```python
from build123d import *

# Parameters (mm, degrees)
SKETCH1_W           = 380
SKETCH1_H           = 179
BOSS_EXTRUDE1_DEPTH = 20
SKETCH2_W           = 20
SKETCH2_H           = 65
SKETCH2_H_2         = 10
CUT_EXTRUDE1_DEPTH  = 20
SKETCH3_R           = 5
CUT_EXTRUDE2_DEPTH  = 159


with BuildPart() as part:
    # Sketch1 → Boss-Extrude1 (new body)
    with BuildSketch(Plane(origin=(0, 0, 0), x_dir=(0, 0, -1), z_dir=(1, 0, 0))):
        Rectangle(SKETCH1_W, SKETCH1_H)
    extrude(amount=BOSS_EXTRUDE1_DEPTH)

    # Sketch2 → Cut-Extrude1 (cut)
    with BuildSketch(Plane.XY.offset(190)):
        with Locations((10, 38)):
            Rectangle(SKETCH2_W, SKETCH2_H)
        with Locations((10, 84.5)):
            Rectangle(SKETCH2_W, SKETCH2_H_2)
        with Locations((10, -84.5)):
            Rectangle(SKETCH2_W, SKETCH2_H_2)
        with Locations((10, -37)):
            Rectangle(SKETCH2_W, SKETCH2_H)
    cut_extrude1 = extrude(amount=-CUT_EXTRUDE1_DEPTH, mode=Mode.SUBTRACT)

    # Sketch3 → Cut-Extrude2 (cut)
    with BuildSketch(Plane(origin=(0, 79.5, 0), x_dir=(1, 0, 0), z_dir=(0, 1, 0))):
        with Locations((10, -180)):
            Circle(SKETCH3_R)
    cut_extrude2 = extrude(amount=-CUT_EXTRUDE2_DEPTH, mode=Mode.SUBTRACT)

    # Mirror2: Cut-Extrude1, Cut-Extrude2 across plane
    add(cut_extrude1.mirror(Plane.XY), mode=Mode.SUBTRACT)
    add(cut_extrude2.mirror(Plane.XY), mode=Mode.SUBTRACT)


solid = part.part
```
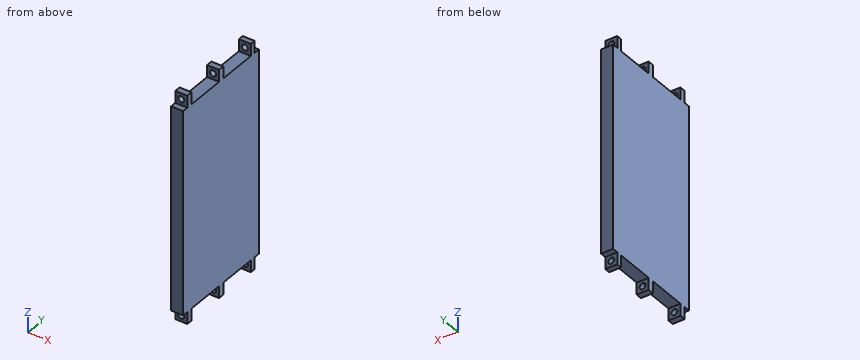
Here's how the part is built. I have some questions about the finished solid (model axes, mm). Coordinates: 2 decimals unless noted, no trailing zeros. Order: outer loops, then holes, each group sorted by start corner. A loop starts at its lowest first (then second) coordinate and runs counter-clockwise, first axis right, second up.
Item 1: I'm going to push flat-ended pins straight in: pin 1 Ø6 at (x, z) = (5, 176.5) entering from +Y; pin 2 Ø6 at (x, z) = (10, 180) entering from -Y; pin 3 Ø5 at (x, y) = (13.5, -83) entering from +Z; pin 4 Ø10 at (x, y) = (18, 23.5) entering from -Z. Where does each tip first touch, or does it pass through?
Response values:
pin 1: stops at y = 79.5
pin 2: passes through
pin 3: stops at z = 170
pin 4: stops at z = -170
Item 2: If we section it at C-C, the plane x = 10: Give the number of separate pieces and of enclosed holes in the cut face, then the cut area to 3 significant figures.
Response values:
separate pieces: 7
enclosed holes: 0
area: 61,400 mm2
Item 3: I need wall thicknesses on probe 1 along Z at (x, y) = (10, -0.5); probe 2 along X at (y, z) = (74, -180); probe 3 along Z at (x, y) = (7, -30.5). Which ranges of each line are inside material? Lowest first, please.
Response values:
probe 1: z = -190 to -185, -175 to 175, 185 to 190
probe 2: x = 0 to 5, 15 to 20
probe 3: z = -170 to 170
Item 4: If we section it at A-A, the plane z = 180: List the corners of the cut face in (x, y) for me, then the cut area to 3 significant figures.
Response values:
outline: (0, -79.5) - (5, -79.5) - (5, -69.5) - (0, -69.5) - close; (0, -4.5) - (5, -4.5) - (5, 5.5) - (0, 5.5) - close; (0, 70.5) - (5, 70.5) - (5, 79.5) - (0, 79.5) - close; (15, -79.5) - (20, -79.5) - (20, -69.5) - (15, -69.5) - close; (15, -4.5) - (20, -4.5) - (20, 5.5) - (15, 5.5) - close; (15, 70.5) - (20, 70.5) - (20, 79.5) - (15, 79.5) - close
area: 290 mm2
Item 5: If we section it at D-D, the plane y = -53.5: List the corners of the cut face in (x, z) for me, then the cut area to 3 significant figures.
Response values:
outline: (0, -170) - (20, -170) - (20, 170) - (0, 170) - close
area: 6,800 mm2
Item 6: If we section it at B-B, the plane y = -1: List the corners of the cut face in (x, z) for me.
Response values:
outline: (0, -190) - (20, -190) - (20, 190) - (0, 190) - close; hole circle Ø10 at (10, -180); hole circle Ø10 at (10, 180)
